from build123d import *

# Parameters (mm, degrees)
SKETCH1_R           = 2.5
BOSS_EXTRUDE1_DEPTH = 14
CUT_EXTRUDE1_DEPTH  = 2
CHAMFER1_SIZE       = 0.2
FILLET1_R           = 0.5


with BuildPart() as part:
    # Sketch1 → Boss-Extrude1 (new body)
    with BuildSketch(Plane(origin=(0, 0, 0), x_dir=(1, 0, 0), z_dir=(0, 1, 0))):
        with Locations(Location((0, 0, 0), (0, 0, 270))):
            Circle(SKETCH1_R)
    extrude(amount=BOSS_EXTRUDE1_DEPTH)

    # Sketch2 → Revolve1 (revolve)
    with BuildSketch(Plane.XY, mode=Mode.PRIVATE) as revolve1_sk:
        Polygon((-5, 16.5), (-2.5, 14), (0, 14), (0, 16.5), align=None)
    revolve(revolve1_sk.sketch.rotate(Axis((0, 14, 0), (0, 1, 0)), 90), axis=Axis((0, 14, 0), (0, 1, 0)))

    # Sketch3 → Cut-Extrude1 (cut)
    with BuildSketch(Plane(origin=(0, 16.5, 0), x_dir=(1, 0, 0), z_dir=(0, 1, 0))):
        Polygon((2, 0), (1, 1.732050808), (-1, 1.732050808), (-2, 0), (-1, -1.732050808), (1, -1.732050808), align=None)
    extrude(amount=-CUT_EXTRUDE1_DEPTH, mode=Mode.SUBTRACT)

    # Chamfer1
    chamfer1_edges = [part.edges().sort_by_distance(p)[0] for p in [
        (1.5, 16.5, 0.866025404),
        (1.5, 16.5, -0.866025404),
        (0, 16.5, -1.732050808),
        (-1.5, 16.5, -0.866025404),
        (-1.5, 16.5, 0.866025404),
        (0, 16.5, 1.732050808),
    ]]
    chamfer(chamfer1_edges, length=CHAMFER1_SIZE)

    # Fillet1
    fillet1_edges = [part.edges().sort_by_distance(p)[0] for p in [
        (0, 14, -2.5),
    ]]
    fillet(fillet1_edges, radius=FILLET1_R)


solid = part.part
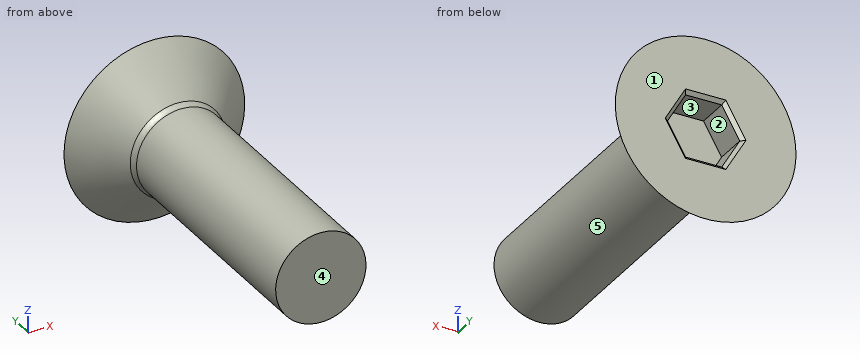
Read the model definition and answer for the solid it produces. Units are mm, in the model's axes. Face numbers are marked on the shaded views. A direction names the side the tool comes from. Round coordinates to 2 decimals unless told otherwise and drop trailing zeros. Write each loop counter-clockwise with the first axis right and the second up, starting at its lowest first coordinate (ties: lowest second). Pieces come first, ordered by that corner, then holes. Notation, with made-up numbers: M 6,-27 L 33,-27 A21 cw 33,-16 Z; hole C 47.25,76 d1. An arc over 180 degrees is marked long. Use a Markdown table: item, result.
1) Straight lines are drawn through the part: line 1 along X through (y, z) = (1.75, -1.5); line 2 along Y through (x, z) = (0.5, -1); line 3 along X through (y, z) = (7.75, 0). For each, find the intervals that lie inside material, in ascending order. Write a range as [from, to].
Answers follow:
| item | result |
|---|---|
| line 1 | x = [-2, 2] |
| line 2 | y = [0, 14.5] |
| line 3 | x = [-2.5, 2.5] |
2) For a pull along X with two mould halves and no side action, classify the marked faces 3, 4 and 5 as pulls with the +X half, pulls with the -X half, needs draft (parallel to the pull), parting line crosses it, or undercut.
Answers follow:
| item | result |
|---|---|
| face 3 | undercut |
| face 4 | needs draft |
| face 5 | parting line crosses it |
3) The part is cut by section A-A (y = 15.5). Write down the section's boundary in (x, z), plus the area to 3 significant figures.
Answers follow:
| item | result |
|---|---|
| outline | C 0,0 d8; hole M -2,0 L -1,-1.73 L 1,-1.73 L 2,0 L 1,1.73 L -1,1.73 Z |
| area | 39.9 mm2 |
4) A tool of negligible diameter and unlimited length cuts with its end or side. For the marked faces 1 and 2, from which of +Z, -Z, +X, -X, +Y, -Y can it reach the whole face along a straight path? Write none if from no direction.
Answers follow:
| item | result |
|---|---|
| face 1 | +Z, -Z, +X, -X, +Y |
| face 2 | +Y |
5) Flat-ended cylindrical pins translate along their axes: pin 1 (2 mm diameter, centred on x = -3, y = 2.5, fed in from +Z); pin 2 (5 mm diameter, centred on x = 3, y = 8.5, fed in from -Z); pin 3 (1 mm diameter, centred on y = 12.5, z = -2.5, fed in from -X). Find the tip coordinate at first contact, or state that the pin passes through.
Answers follow:
| item | result |
|---|---|
| pin 1 | stops at z = 1.5 |
| pin 2 | stops at z = -2.45 |
| pin 3 | stops at x = -1.5 |
6) The part is cut by section B-B (y = 5). Write down the section's boundary in (x, z), plus the area to 3 significant figures.
Answers follow:
| item | result |
|---|---|
| outline | C 0,0 d5 |
| area | 19.6 mm2 |
